Verification items for this drawing (mm, ordinates from the low corner). Round coordinates to 2 decimals unless told otherwise and drop trailing zeros. Write each loop counter-clockwise with the first axis right and the second up, starting at its lowest first coordinate (ties: lowest second). Pieces come first, ordered by that corner, then holes. Notation, with made-up numbers: (11, -3) -> (58, -3) arc R24 cw to (58, 18) -> close; hole circle Ø11 at (-5, 68). An arc over 180 degrees is marked (long way). One line per question, with ' | ' between items.
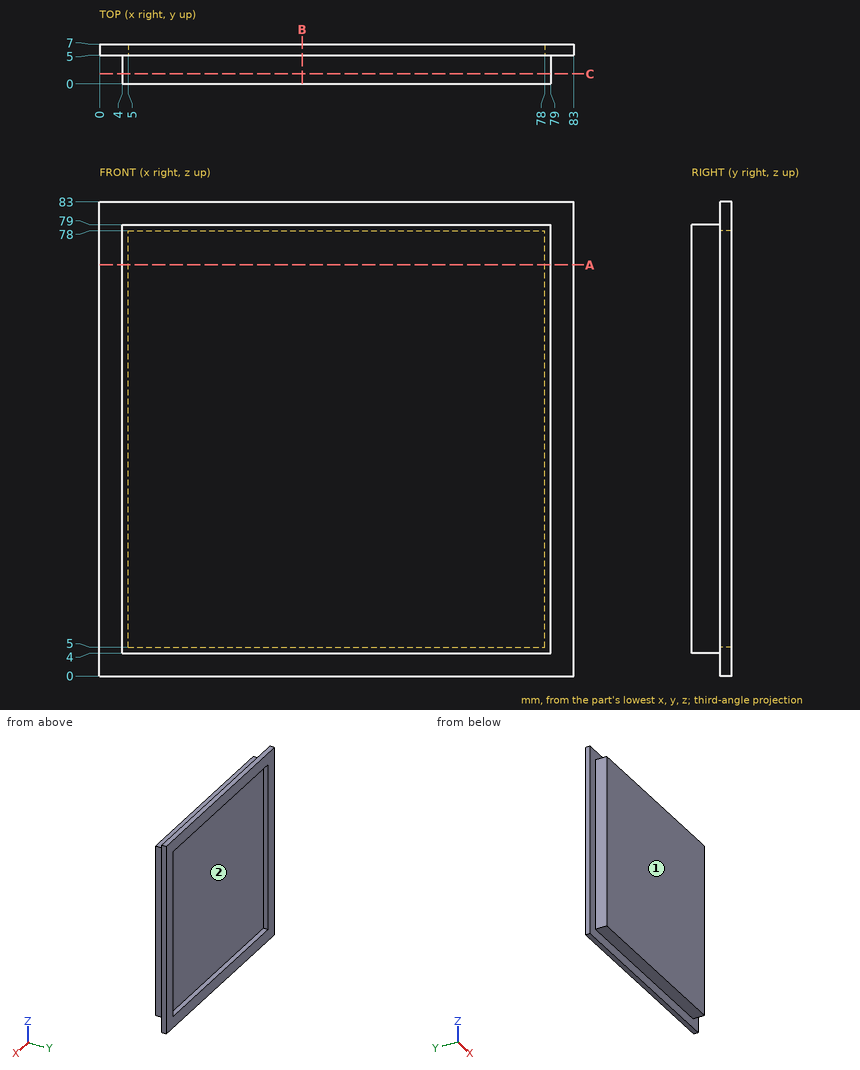
(1) Sectioned sample at B-B on x = 35.5. Record the cut outline in (y, z), then the cut area to 3 significant figures.
Resolved:
outline: (0, 4) -> (5, 4) -> (5, 0) -> (7, 0) -> (7, 5) -> (5, 5) -> (5, 78) -> (7, 78) -> (7, 83) -> (5, 83) -> (5, 79) -> (0, 79) -> close | area: 395 mm2
(2) Sectioned sample at A-A on z = 72. Record the cut outline in (x, y), then the cut area to 3 significant figures.
Resolved:
outline: (0, 5) -> (4, 5) -> (4, 0) -> (79, 0) -> (79, 5) -> (83, 5) -> (83, 7) -> (78, 7) -> (78, 5) -> (5, 5) -> (5, 7) -> (0, 7) -> close | area: 395 mm2
(3) Material ranges on line 1 (Z direction, x = 44, y = 5.75); line 2 (Y direction, x = 22, z = 5.5); line 3 (Z direction, x = 16, y = 4.75), recorded low to high.
Resolved:
line 1: z = 0 to 5, 78 to 83 | line 2: y = 0 to 5 | line 3: z = 4 to 79
(4) Go/stop test with flat-tipped pins: pin 1 (4 mm diameter, centred on x = 47.5, z = 25.5, fed in from +Y); pin 2 (2.5 mm diameter, centred on x = 55, y = 2, fed in from +Z); pin 3 (1.5 mm diameter, centred on y = 2, z = 46, fed in from +X); pin 4 (10 mm diameter, centred on x = 47.5, z = 13, fed in from -Y). Record where each tip stops, or that it passes through.
Resolved:
pin 1: stops at y = 5 | pin 2: stops at z = 79 | pin 3: stops at x = 79 | pin 4: stops at y = 0
(5) Draft check along X on the marked faces 1 and 2. Enter one of: +X half, -X half, draft (parallel to the pull), parting line (faces both ways), or undercut.
Resolved:
face 1: draft | face 2: undercut
(6) Sectioned sample at C-C on y = 1.75. Record the cut outline in (x, z), then the cut area to 4 significant figures.
Resolved:
outline: (4, 4) -> (79, 4) -> (79, 79) -> (4, 79) -> close | area: 5,625 mm2
